Geometry: see drawing. Coordinates: mm, zero at the bounding-box minimum. Coordinates: 2 decimals unless noted, no trailing zeros. Write each loop counter-clockwise with the first axis right and the second up, starting at its lowest first coordinate (ties: lowest second). Pieces come first, ordered by that corner, then holes.
1) Line query: L1, parallel to X at y = 9.5, z = 14.5; L2, parallel to X at y = 11, z = 24.5 (1 decimal). Output: solid intervals per line, ascending.
2) Section query B-B (x = 10.5). Output: boundary loops of the cut face in (y, z).
3) Draft query along X for the marked faces 1, 2 and 3. Return one class per face: pulls with the +X half, pulls with the -X half, needs draft (parallel to the pull), parting line crosses it, or undercut.
4) Section query A-A (y = 34.5). Output: boundary loops of the cut face in (x, z) (1 decimal), then the cut area to 3 significant figures.
5) Section query C-C (z = 18.5). State how many separate pieces and enclosed holes the cut face has, then the cut area to 4 significant figures.
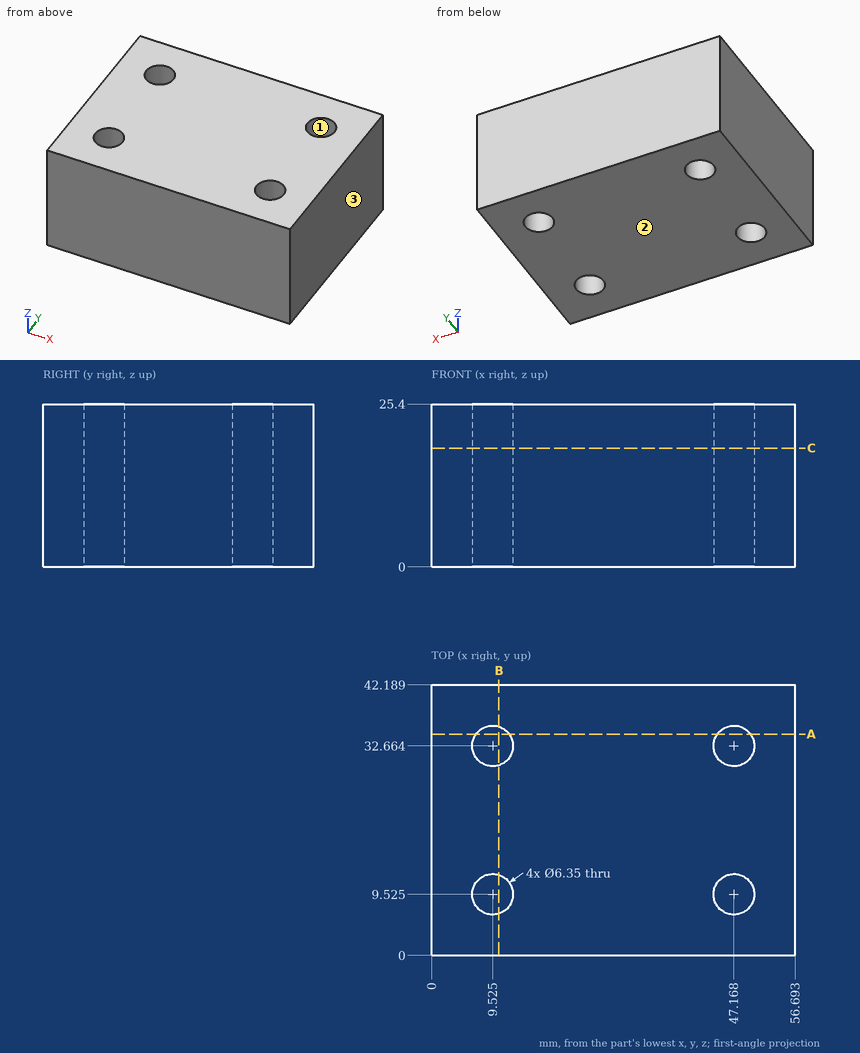
Answer:
1. L1: x = 0 to 6.35, 12.7 to 43.99, 50.34 to 56.69
1. L2: x = 0 to 6.7, 12.3 to 44.4, 50 to 56.7
2. outline: (0, 0) - (6.5, 0) - (6.5, 25.4) - (0, 25.4) - close; (12.55, 0) - (29.64, 0) - (29.64, 25.4) - (12.55, 25.4) - close; (35.69, 0) - (42.19, 0) - (42.19, 25.4) - (35.69, 25.4) - close
3. face 1: undercut
3. face 2: needs draft
3. face 3: pulls with the +X half
4. outline: (0, 0) - (6.9, 0) - (6.9, 25.4) - (0, 25.4) - close; (12.1, 0) - (44.6, 0) - (44.6, 25.4) - (12.1, 25.4) - close; (49.8, 0) - (56.7, 0) - (56.7, 25.4) - (49.8, 25.4) - close
4. area: 1,180 mm2
5. separate pieces: 1
5. enclosed holes: 4
5. area: 2,265 mm2
